Could you check a few things on this model? Use its own coordinates, in mm. Face numbers are marked on the shaded views. A direction names the side the tool comes from. Give positions to 0.01 mm unless a question says otherwise; leave off trailing zeros. Loops run counter-clockwise (first coordinate to the right, second up) from the corner with the lowest first, then second, coordinate; pieces in that order, holes last. Notation, with made-up numbers: M 28.5,72.5 L 52.5,72.5 A31 ccw 52.5,98.5 Z; hole C 61.25,70.25 d11. An arc over 180 degrees is marked long. Use CSV: the item, a comma, the result in double quotes.
Autodesk Inventor part; units mm, degrees
ref_plane "YZ Plane" through (0, 0, 0) normal (1, 0, 0) x (0, 1, 0)
ref_plane "XZ Plane" through (0, 0, 0) normal (0, 1, 0) x (-1, 0, 0)
ref_plane "XY Plane" through (0, 0, 0) normal (0, 0, 1) x (1, 0, 0)
sketch "Sketch2" plane through (0, 0, 0) normal (0, 1, 0) x (-1, 0, 0)
  circle A0 centre (0, 0) radius 22
  circle A1 centre (0, 0) radius 30
  dimension "d0" = 44
  dimension "d1" = 60
extrude "Extrusion1" add sketch "Sketch2" along normal blind 10
sketch "Sketch3" plane through (0, 10, 0) normal (0, 1, 0) x (1, 0, 0)
  circle A0 centre (0, 0) radius 30
  circle A1 centre (0, 0) radius 15
  dimension "d4" = 30
extrude "Extrusion2" add sketch "Sketch3" along normal blind 5
sketch "Sketch4" plane through (0, 15, 0) normal (0, 1, 0) x (1, 0, 0)
  circle A0 centre (0, 0) radius 15
  circle A1 centre (0, 0) radius 19
  dimension "d7" = 38
  dimension "d8" = 30
extrude "Extrusion3" add sketch "Sketch4" along normal blind 10
properties part number "smallbearingcup" material "Steel"
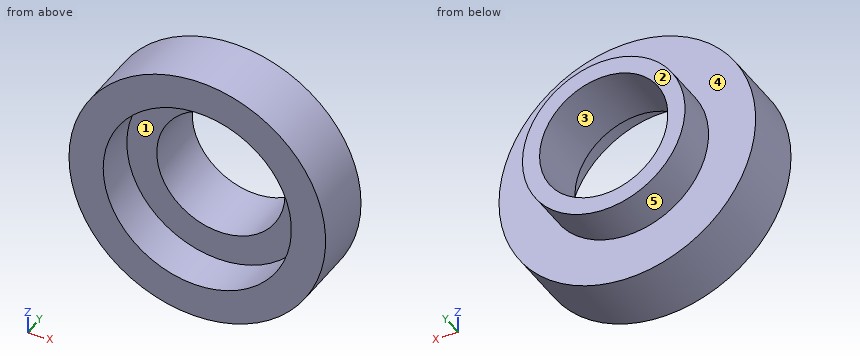
1. I'm going to push flat-ended pins straight in: pin 1 Ø1.5 at (x, z) = (-14.5, -1.5) entering from -Y; pin 2 Ø1 at (y, z) = (13, -10.5) entering from -X; pin 3 Ø8 at (x, y) = (3, 21) entering from +Z. Where does each tip first touch, or does it pass through?
Outcome:
pin 1,"y = 10"
pin 2,"x = -28.28"
pin 3,"z = 19"
2. Please list where these lines run through material, in increasing order: line 1 (X direction, y = 18.25, z = 0); line 2 (Z direction, x = 0, y = 3.25).
Outcome:
line 1,"-19 to -15, 15 to 19"
line 2,"-30 to -22, 22 to 30"
3. Which directions (+Z, -Z, +X, -X, +Y, -Y) give clear straight access to the entire face, cutting with the end or side of a thin tool? Please do the marked faces 1 and 2.
Outcome:
face 1,"-Y"
face 2,"+Z, -Z, +X, -X, +Y"
4. If we mould it in two halves opening along Z, with no side actions, what happens to the marked faces 3, 4 and 5? For each: +Z half, -Z half, draft (parallel to the pull), parting line (faces both ways), or undercut.
Outcome:
face 3,"undercut"
face 4,"draft"
face 5,"parting line"
5. I want a section at D-D, the plane z = -18. List the corners of the cut face in (x, y) for me.
Outcome:
outline,"M -24,0 L -12.65,0 L -12.65,10 L 12.65,10 L 12.65,0 L 24,0 L 24,15 L 6.08,15 L 6.08,25 L -6.08,25 L -6.08,15 L -24,15 Z"
6. I want a section at C-C, the plane y = 21.25. List the corners of the cut face in (x, z) for me, then the cut area to 3 significant figures.
Outcome:
outline,"C 0,0 d38; hole C 0,0 d30"
area,"427 mm2"
7. I want a section at B-B, the plane z = -2. List the corners of the cut face in (x, y) for me.
Outcome:
outline,"M -29.93,0 L -21.91,0 L -21.91,10 L -14.87,10 L -14.87,25 L -18.89,25 L -18.89,15 L -29.93,15 Z; M 14.87,10 L 21.91,10 L 21.91,0 L 29.93,0 L 29.93,15 L 18.89,15 L 18.89,25 L 14.87,25 Z"
